Check sheet for the drawn part. Datum: minimum x, y, z corner. Units: mm. A direction names the side the tool comes from. Round coordinates to 2 decimals unless told otherwise and drop trailing zeros. Loops run counter-clockwise (first coordinate to the right, second up) from the corner with the lowest first, then second, coordinate; pieces in that order, holes last.
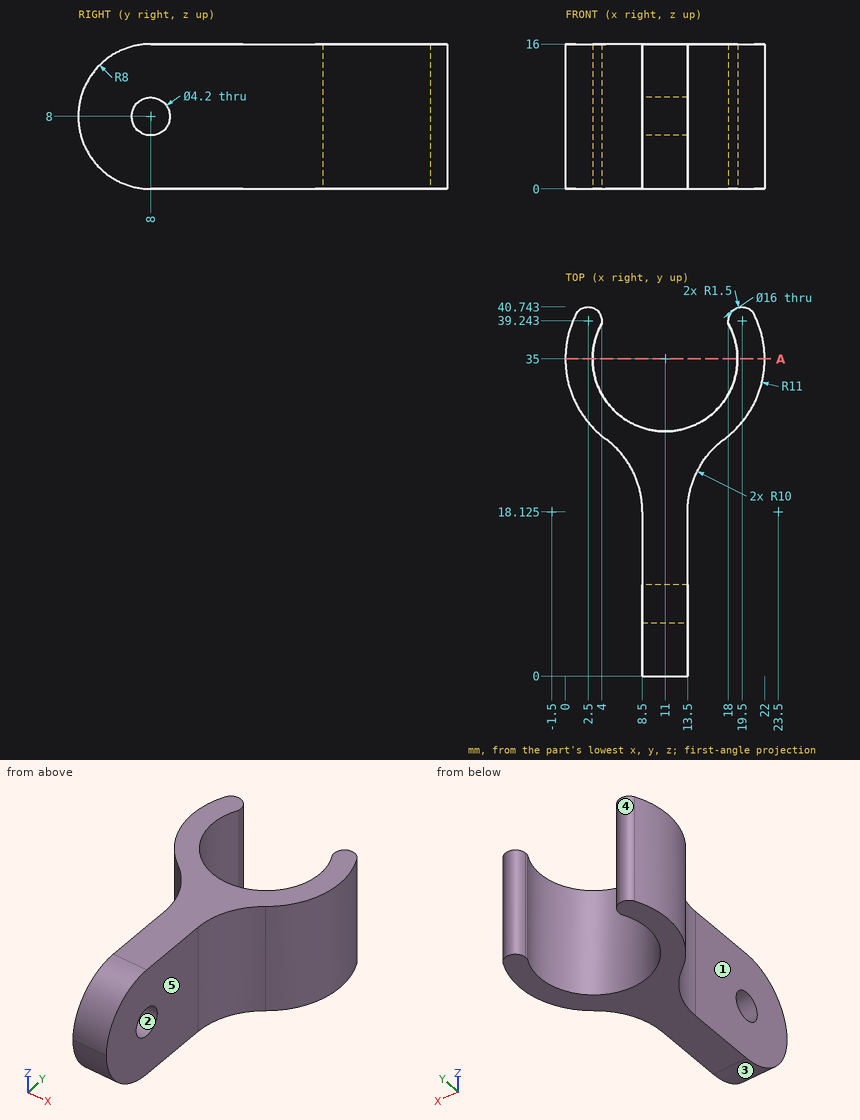
1) Mould release check, pull along Y, two halves, no side actions. Record for the marked faces 1, 2 and 3: +Y half, -Y half, draft (parallel to the pull), parting line (faces both ways), or undercut.
Report:
face 1: draft
face 2: undercut
face 3: -Y half
2) Access from +Z, -Z, +X, -X, +Y, -Y to the whole of each face (thin tool, end or side, straight path). Record for the marked faces 4 and 5.
Report:
face 4: +Z, -Z, +Y
face 5: +Z, -Z, +X, -Y
3) Sectioned sample at A-A, the plane y = 35. Record the cut outline in (x, z).
Report:
outline: (0, 0) - (3, 0) - (3, 16) - (0, 16) - close; (19, 0) - (22, 0) - (22, 16) - (19, 16) - close
4) Gauge pin test, flat ends, axial feed: pin 1 (3 mm diameter, centred on y = 31, z = 14, fed in from +X); pin 2 (5.5 mm diameter, centred on y = 8, z = 8, fed in from +X); pin 3 (5 mm diameter, centred on x = 12.5, z = 4, fed in from -Y); pin 4 (5 mm diameter, centred on x = 7, y = 32.5, fed in from -Z). Record the tip position at first contact, or that the pin passes through.
Report:
pin 1: stops at x = 21.71
pin 2: stops at x = 13.5
pin 3: stops at y = 0.14
pin 4: passes through
5) Scan lines: line 1 along Z through (x, y) = (11.8, 8); line 2 along X through (y, z) = (18.5, 1.75); line 3 along X through (y, z) = (31, 9.75) (1 decimal). Record each from-to range of solid material in increasing order.
Report:
line 1: z = 0 to 5.9, 10.1 to 16
line 2: x = 8.49 to 13.51
line 3: x = 0.8 to 4.1, 17.9 to 21.2
